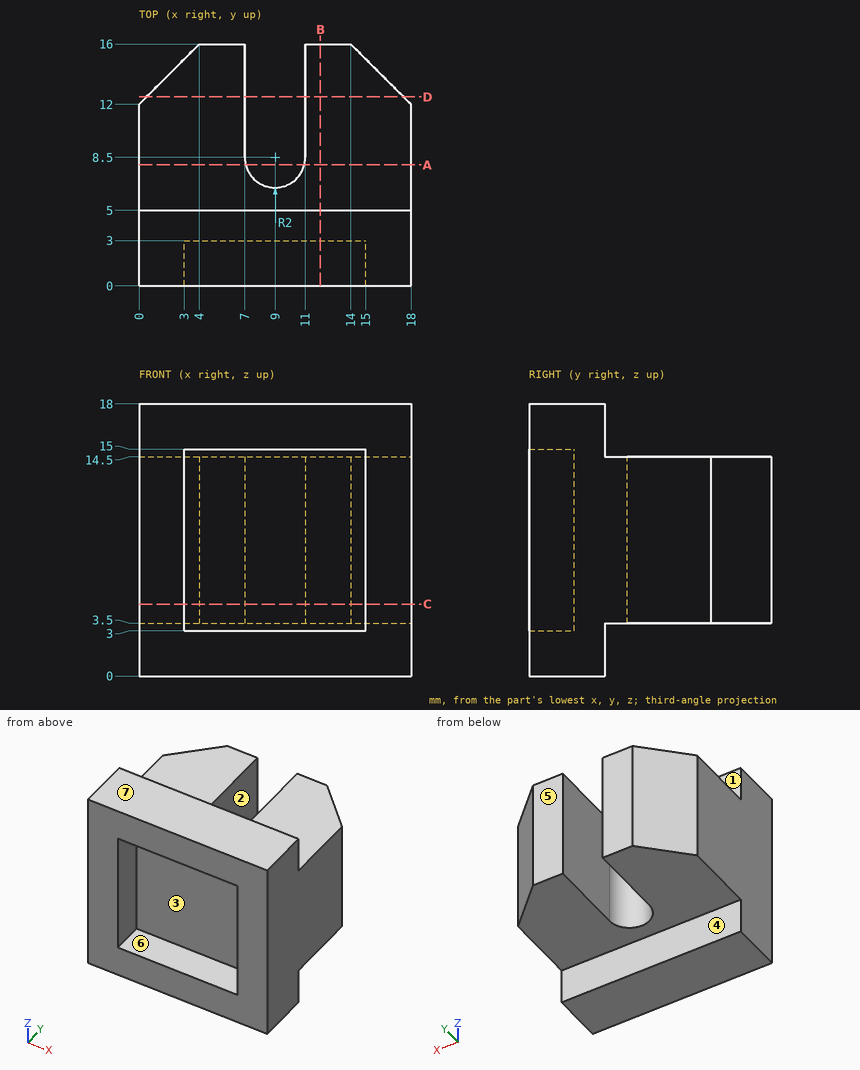
Print and shaded views of the part. All mm, measured from the part's lowest x, y and z. A direction names the side the tool comes from. Round coordinates to 2 decimals unless told otherwise and drop trailing zeros. Write each loop counter-clockwise with the first axis right and the second up, starting at its lowest first coordinate (ties: lowest second). Pieces come first, ordered by that corner, then holes. Notation, with made-up numbers: (-21, -21.75) -> (38, -21.75) arc R25 ccw to (38, 5.25) -> close; hole circle Ø11 at (16.25, 47). An arc over 180 degrees is marked (long way). Answer in a Markdown table with one row per item. Add a question column.
Item 1: Drop flat-ended pins along their axis: pin 1 Ø3.5 at (x, y) = (8, 13) entering from +Z; pin 2 Ø1.5 at (y, z) = (14, 16) entering from -X; pin 3 Ø9 at (x, y) = (6.5, 10.5) entering from -Z; pin 4 Ø3 at (x, z) = (10, 16.5) entering from +Y. Give the stop position or say it passes through.
Item 2: Drill centre lines: line 1 (X direction, y = 1.75, z = 14.25); line 2 (Z direction, x = 1, y = 9.25). Where is each one in solid material? Low to high. Write a range as from..to.
Item 3: Saw through at B-B, the plane x = 12. Write the cut outline in (y, z), then the cut area to 3 significant figures.
Item 4: Saw through at D-D, the plane y = 12.5. Write the cut outline in (x, z).
Item 5: Mould opens along Z. For the marked faces 5, 6 and 7 say: pulls with the +Z half, pulls with the -Z half, needs draft (parallel to the pull), parting line crosses it, or undercut.
Item 6: Which spindle directions (+Z, -Z, +X, -X, +Y, -Y) get a long thin tool onto all of the face, cutting with end or side? Do the marked faces 1, 2, 3 and 4. Say none if no direction does.
Item 7: Saw through at A-A, the plane y = 8. Write the cut outline in (x, z), then the cut area to 3 significant figures.
Item 8: Saw through at C-C, the plane z = 4.75. Write the cut outline in (x, y).
Findings below:
| question | item | result |
|---|---|---|
| 1 | pin 1 | stops at z = 14.5 |
| 1 | pin 2 | passes through |
| 1 | pin 3 | stops at z = 3.5 |
| 1 | pin 4 | stops at y = 5 |
| 2 | line 1 | x = 0..3, 15..18 |
| 2 | line 2 | z = 3.5..14.5 |
| 3 | outline | (0, 0) -> (5, 0) -> (5, 3.5) -> (16, 3.5) -> (16, 14.5) -> (5, 14.5) -> (5, 18) -> (0, 18) -> (0, 15) -> (3, 15) -> (3, 3) -> (0, 3) -> close |
| 3 | area | 175 mm^2 |
| 4 | outline | (0.5, 3.5) -> (7, 3.5) -> (7, 14.5) -> (0.5, 14.5) -> close; (11, 3.5) -> (17.5, 3.5) -> (17.5, 14.5) -> (11, 14.5) -> close |
| 5 | face 5 | needs draft |
| 5 | face 6 | undercut |
| 5 | face 7 | pulls with the +Z half |
| 6 | face 1 | +Z, +X, -X, +Y |
| 6 | face 2 | +Z, -Z, +Y |
| 6 | face 3 | -Y |
| 6 | face 4 | -Z, +X, -X, +Y |
| 7 | outline | (0, 3.5) -> (7.06, 3.5) -> (7.06, 14.5) -> (0, 14.5) -> close; (10.94, 3.5) -> (18, 3.5) -> (18, 14.5) -> (10.94, 14.5) -> close |
| 7 | area | 155 mm^2 |
| 8 | outline | (0, 0) -> (3, 0) -> (3, 3) -> (15, 3) -> (15, 0) -> (18, 0) -> (18, 12) -> (14, 16) -> (11, 16) -> (11, 8.5) arc R2 cw to (7, 8.5) -> (7, 16) -> (4, 16) -> (0, 12) -> close |
